The model under review builds one solid part; all positions refer to its coordinate system, in mm. Face numbers are marked on the shaded views. Round coordinates to 2 decimals unless told otherwise and drop trailing zeros. Loops run counter-clockwise (first coordinate to the right, second up) from the corner with the lowest first, then second, coordinate; pieces in that order, holes last. Notation, with made-up numbers: (43.5, 67.5) -> (57.5, 67.5) arc R29 cw to (57.5, 98.5) -> close; hole circle Ø9 at (80.25, 16). An arc over 180 degrees is marked (long way). Use CSV: the item, a comma, the result in double quotes. Start each with the question number.
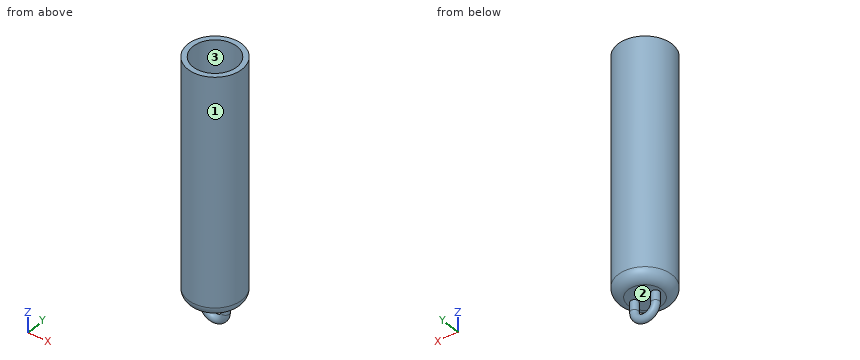
```python
from build123d import *

# Parameters (mm, degrees)
ESQUISSE2_R        = 10.65
ESQUISSE2_R_2      = 8.65
BOSS_EXTRU_1_DEPTH = 45
ESQUISSE5_R        = 1.5


with BuildPart() as part:
    # Esquisse2 → Boss.-Extru.1 (new, symmetric)
    with BuildSketch(Plane.XY):
        with Locations(Location((0, 0, 0), (0, 0, 180))):
            Circle(ESQUISSE2_R)
        with Locations(Location((0, 0, 0), (0, 0, 180))):
            Circle(ESQUISSE2_R_2, mode=Mode.SUBTRACT)
    extrude(amount=BOSS_EXTRU_1_DEPTH, both=True)

    # Esquisse3 → Révolution1 (revolve)
    with BuildSketch(Plane(origin=(0, 0, 0), x_dir=(1, 0, 0), z_dir=(0, 1, 0))):
        with BuildLine():
            Line((-6.65, 49), (0, 49))
            Line((0, 49), (0, 45))
            Line((0, 45), (-10.65, 45))
            ThreePointArc((-10.65, 45), (-9.478427125, 47.828427125), (-6.65, 49))
        make_face()
    revolve(axis=Axis((0, 0, -49), (0, 0, 1)))

    # Balayage3: sweep along a path in Esquisse6
    with BuildLine(Plane(origin=(0, 0, 0), x_dir=(1, 0, 0), z_dir=(0, 1, 0))) as balayage3_path:
        Line((-2.65, 45), (-2.65, 52.85))
        ThreePointArc((-2.65, 52.85), (0, 55.5), (2.65, 52.85))
        Line((2.65, 52.85), (2.65, 45))
    # Esquisse5 → Balayage3 (sweep)
    with BuildSketch(Plane(origin=(0, 0, 0), x_dir=(0, 0, -1), z_dir=(1, 0, 0))):
        with Locations((57, 0)):
            Circle(ESQUISSE5_R)
    sweep(path=balayage3_path.line)


solid = part.part
```
1. The part is to be moulded in two halves that separate along Y. For the marked faces 1, 2 and 3, say which applies: pulls with the +Y half, pulls with the -Y half, needs draft (parallel to the pull), parting line crosses it, or undercut.
2. Clearance check with flat-ended pins moving along their axes: P1, Ø1, axis at x = 0, y = -1.5, coming from the -Z side; P2, Ø12, axis at x = -4, y = -5, coming from the -Z side; P3, Ø8, axis at y = 3.5, z = 28, coming from the -X side; P4, Ø4, axis at x = -7, z = 33, coming from the +Y side. State where each tip first meets the part, or that it passes through.
3. Take a section at C-C, the plane z = -11. Give the boundary of the cut face in (x, y), then the cut area to 3 significant figures.
4. For line 1 along Y through (x, z) = (0, 12.5); line 2 along Y through (x, z) = (1.5, -9); line 3 along X through (y, z) = (2.5, -14), list the stretches that pass through material, from the lowest coordinate up. Write a range as from..to.
5. Take a section at B-B, the plane x = 0. Give the boundary of the cut face in (y, z), then the cut area to 3 significant figures.
6. Take a section at A-A, the plane y = 0. Give the boundary of the cut face in (x, z).
Results:
1,face 1,"parting line crosses it"
1,face 2,"needs draft"
1,face 3,"undercut"
2,P1,"z = -58.12"
2,P2,"z = -58.47"
2,P3,"x = -10.65"
2,P4,"y = 9.4"
3,outline,"circle Ø21.3 at (0, 0); hole circle Ø17.3 at (0, 0)"
3,area,"121 mm²"
4,line 1,"-10.65..-8.65, 8.65..10.65"
4,line 2,"-10.54..-8.52, 8.52..10.54"
4,line 3,"-10.35..-8.28, 8.28..10.35"
5,outline,"(-10.65, -45) arc R4 ccw to (-6.65, -49) -> (6.65, -49) arc R4 ccw to (10.65, -45) -> (10.65, 45) -> (8.65, 45) -> (8.65, -45) -> (-8.65, -45) -> (-8.65, 45) -> (-10.65, 45) -> close; circle Ø3 at (0, -57)"
5,area,"445 mm²"
6,outline,"(-10.65, -45) arc R4 ccw to (-6.65, -49) -> (-5.65, -49) -> (-5.65, -52.85) arc R5.65 ccw to (5.65, -52.85) -> (5.65, -49) -> (6.65, -49) arc R4 ccw to (10.65, -45) -> (10.65, 45) -> (8.65, 45) -> (8.65, -45) -> (-8.65, -45) -> (-8.65, 45) -> (-10.65, 45) -> close; hole (-2.65, -52.85) arc R2.65 ccw to (2.65, -52.85) -> (2.65, -49) -> (-2.65, -49) -> close"
